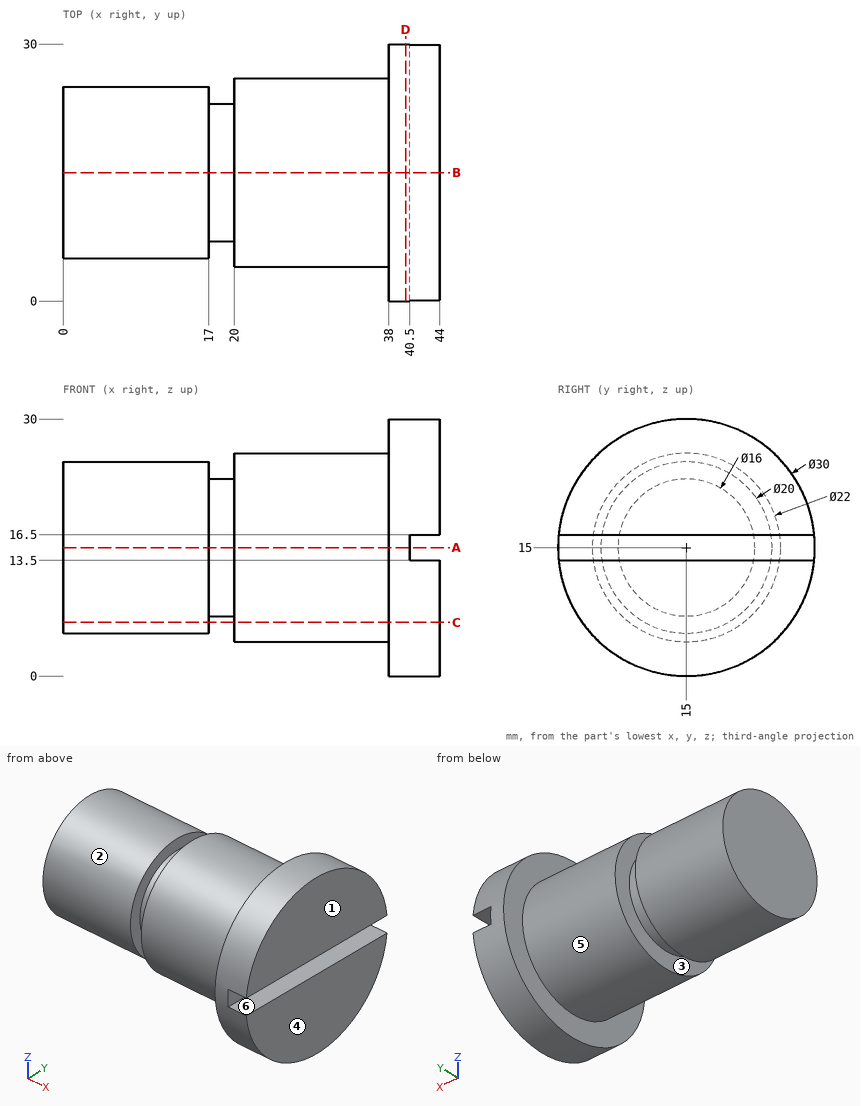
Verification items for this drawing (mm, ordinates from the low corner). A direction names the side the tool comes from. Coordinates: 2 decimals unless noted, no trailing zeros. Write each loop counter-clockwise with the first axis right and the second up, starting at its lowest first coordinate (ties: lowest second). Pieces come first, ordered by that corner, then holes. Notation, with made-up numbers: M 41,45 L 62,45 A13 ccw 62,70 Z; hole C 34,-13 d3. An arc over 180 degrees is marked long. Answer as a JSON object with one key per item and string values. Group by question number.
(1) Release check for a two-part mould opening along Z. For the marked faces 4, 5 and 6 record: +Z half, -Z half, draft (parallel to the pull), parting line (faces both ways), or undercut.
(2) Cross-section at D-D, the plane x = 40. Record the cut outline in (y, z).
(3) Tool access check on the marked faces 1, 2 and 3. Record the directions out of +Z, -Z, +X, -X, +Y, -Y that give a thin tool (end or side, any length) a straight path to the whole face; none if there is none.
(4) Cross-section at A-A, the plane z = 15. Record the cut outline in (x, y), and give its area (3 significant figures).
(5) Gauge pin test, flat ends, axial feed: pin 1 (4 mm diameter, centred on x = 43, y = 19.5, fed in from +Z); pin 2 (4 mm diameter, centred on x = 42, y = 12, fed in from -Z); pin 3 (8 mm diameter, centred on x = 33.5, z = 24, fed in from -Y). Record the tip position at first contact, or that the pin passes through.
(6) Material ranges on line 1 (X direction, y = 17.25, z = 14); line 2 (X direction, y = 1.5, z = 10.25); line 3 (X direction, y = 5.25, z = 15.25), recorded low to high.
(7) Cross-section at C-C, the plane z = 6.25. Record the cut outline in (x, y).
(8) Cross-section at B-B, the plane y = 15. Record the cut outline in (x, z), and give its area (4 significant figures).
Reply:
{
 "1": {"face 4": "draft", "face 5": "parting line", "face 6": "undercut"},
 "2": {"outline": "C 15,15 d30"},
 "3": {"face 1": "+Z, -Z, +X, +Y, -Y", "face 2": "-X", "face 3": "none"},
 "4": {"outline": "M 0,5 L 17,5 L 17,7 L 20,7 L 20,4 L 38,4 L 38,0 L 40.5,0 L 40.5,30 L 38,30 L 38,26 L 20,26 L 20,23 L 17,23 L 17,25 L 0,25 Z", "area": "859 mm²"},
 "5": {"pin 1": "z = 29.79", "pin 2": "z = 0.03", "pin 3": "y = 5.2"},
 "6": {"line 1": "0 to 40.5", "line 2": "38 to 44", "line 3": "0 to 17, 20 to 40.5"},
 "7": {"outline": "M 0,10.16 L 17,10.16 L 17,19.84 L 0,19.84 Z; M 20,8.33 L 38,8.33 L 38,2.82 L 44,2.82 L 44,27.18 L 38,27.18 L 38,21.67 L 20,21.67 Z"},
 "8": {"outline": "M 0,5 L 17,5 L 17,7 L 20,7 L 20,4 L 38,4 L 38,0 L 44,0 L 44,13.5 L 40.5,13.5 L 40.5,16.5 L 44,16.5 L 44,30 L 38,30 L 38,26 L 20,26 L 20,23 L 17,23 L 17,25 L 0,25 Z", "area": "953.5 mm²"}
}
